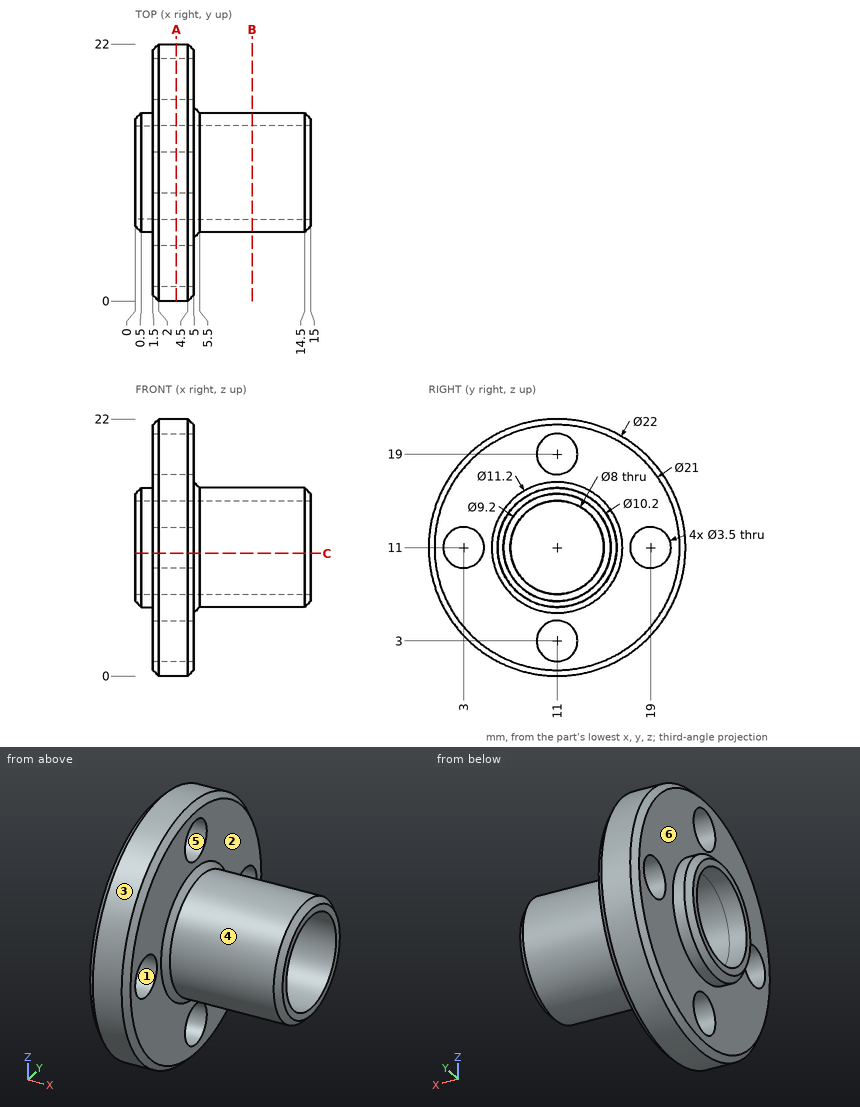
Could you check a few things on this drawing? It's one solid part, dimensions in mm from its lowest x, y, z. A direction names the side the tool comes from. Coordinates: 2 decimals unless noted, no trailing zeros. Order: outer loops, then holes, each group sorted by start corner. A loop starts at its lowest first (then second) coordinate and runs counter-clockwise, first axis right, second up. Notation, with made-up numbers: M 31.25,48.5 L 65.25,48.5 A27 cw 65.25,70.5 Z; hole C -8,-37 d6. An arc over 180 degrees is marked long. Answer as a JSON object with one key per item and string values. Group by question number.
(1) For pin 1 (1 mm diameter, centred on y = 8, z = 2.5, fed in from +X); pin 2 (4 mm diameter, centred on y = 11, z = 19, fed in from -X); pin 3 (5 mm diameter, centred on y = 11, z = 11, fed in from +X); pin 4 (4 mm diameter, centred on y = 13.5, z = 17.5, fed in from +X), each with a flat end and sliding along its axis, tell me the tip position at first contact or that it passes through.
(2) If we mould it in two halves opening along Z, with no side actions, what happens to the marked faces 1, 2 and 3? For each: released by +Z, released by -Z, zero draft, split by the parting line, or undercut.
(3) Suppose I cut it at C-C, the plane z = 10.5. State how many separate pieces and enclosed holes the cut face has, then the cut area to 3 significant figures.
(4) Suppose I cut it at B-B, the plane x = 10. Please give me the cut outline in (y, z), then the cut area to 3 significant figures.
(5) Suppose I cut it at A-A, the plane x = 3.5. Please give me the cut outline in (y, z), then the cut area to 3 significant figures.
(6) I need wall thicknesses on probe 1 along Y at (x, z) = (2.5, 12); probe 2 along X at (y, z) = (16.5, 13.25); probe 3 along Z at (x, y) = (4.75, 9.5). Which ranges of each line are inside material? Lowest first, please.
(7) Which directions (+Z, -Z, +X, -X, +Y, -Y) give clear straight access to the entire face, cutting with the end or side of a thin tool? Please do the marked faces 4, 5 and 6.
Values found:
{
 "1": {"pin 1": "stops at x = 5", "pin 2": "stops at x = 1.5", "pin 3": "passes through", "pin 4": "stops at x = 14.64"},
 "2": {"face 1": "undercut", "face 2": "zero draft", "face 3": "split by the parting line"},
 "3": {"separate pieces": "4", "enclosed holes": "0", "area": "50.4 mm^2"},
 "4": {"outline": "C 11,11 d10.2; hole C 11,11 d8", "area": "31.4 mm^2"},
 "5": {"outline": "C 11,11 d22; hole C 3,11 d3.5; hole C 11,11 d8; hole C 11,3 d3.5; hole C 11,19 d3.5; hole C 19,11 d3.5", "area": "291 mm^2"},
 "6": {"probe 1": "y = 0.05 to 1.56, 4.44 to 7.13, 14.87 to 17.56, 20.44 to 21.95", "probe 2": "x = 1.5 to 5", "probe 3": "z = 0.36 to 2.1, 3.9 to 7.29, 14.71 to 18.1, 19.9 to 21.64"},
 "7": {"face 4": "+X", "face 5": "+X, -X", "face 6": "-X"}
}
